```python
from build123d import *

# Parameters (mm, degrees)
F0_W     = 203.2
F0_H     = 203.2
F1_DEPTH = 9.525
F3_DEPTH = 76.2
F4_W     = 38.1
F4_H     = 63.5
F5_DEPTH = 101.6
F6_W     = 101.6
F6_H     = 190.5
F6_H_2   = 152.4
F7_DEPTH = 53.975


with BuildPart() as f1:
    # F0 (on Front) → F1 (new body, symmetric)
    with BuildSketch(Plane.XZ):
        Rectangle(F0_W, F0_H)
    extrude(amount=F1_DEPTH, both=True)

    # F2 (on Right) → F3 (join, symmetric)
    with BuildSketch(Plane.YZ):
        Polygon((-9.525, -101.6), (-9.525, 165.1), (-63.5, 165.1), (-63.5, 12.7), (-22.225, -101.6), align=None)
    extrude(amount=F3_DEPTH, both=True)

    # F4 (on Right) → F5 (cut, symmetric)
    with BuildSketch(Plane.YZ):
        with Locations((-9.525, 133.35)):
            Rectangle(F4_W, F4_H)
    extrude(amount=F5_DEPTH, both=True, mode=Mode.SUBTRACT)

    # F6 (on face) → F7 (cut, through all)
    with BuildSketch(Plane.XZ.offset(63.5)):
        with Locations((0, -82.55)):
            Rectangle(F6_W, F6_H)
        with Locations((0, 88.9)):
            Rectangle(F6_W, F6_H_2)
    extrude(amount=-F7_DEPTH, mode=Mode.SUBTRACT)


solid = f1.part
```
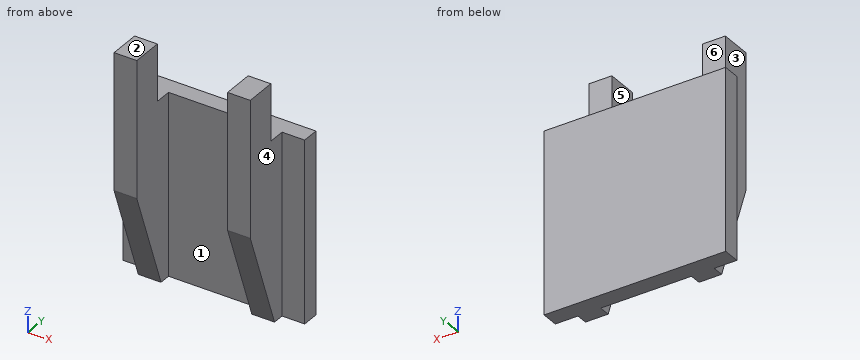
Source: CAD feature listing. Evaluate the final solid. Frame: model axes, mm. Face numbers are marked on the shaded views. A direction names the side the tool comes from. Round coordinates to 2 decimals unless told otherwise and drop trailing zeros. Write each loop counter-clockwise with the first axis right and the second up, starting at its lowest first coordinate (ties: lowest second). Pieces come first, ordered by that corner, then holes. Notation, with made-up numbers: M 42.25,-28.5 L 101.25,-28.5 A17 cw 101.25,-3.5 Z; hole C 5.5,0 d11. An arc over 180 degrees is marked long. Use CSV: the item, a comma, the result in double quotes. Start each with the question number.
Q1. Pull-direction query (X, two-part tool) for the marked faces 1, 2 and 3; classes: +X half, -X half, draft (parallel to the pull), parting line (faces both ways), or undercut.
Q2. Cut plane A-A on y = -15.5. Output: boundary loops of the cut face in (x, z), plus the area to 3 significant figures.
Q3. Line query: line 1 (X direction, y = -17.5, z = 33); line 2 (Y direction, x = 27, z = -9.5) (3 decimals); line 3 (Z direction, x = 50.5, y = -4). Output: solid intervals per line, ascending. Write a range as from..to.
Q4. Cut plane B-B on z = 44.5. Output: boundary loops of the cut face in (x, y) (3 decimals), plus the area to 3 significant figures.
Q5. Access query for the marked faces 4, 5 and 6. Directions: +Z, -Z, +X, -X, +Y, -Y. A direction counts if a zero-diameter tool reaches every point of the face in a straight line with its end or side. Return the directions, or none.
Q6. Cut plane C-C on x = -70. Output: boundary loops of the cut face in (y, z) (3 decimals), plus the area to 3 significant figures.
Q7. Cut plane D-D on y = -42. Output: boundary loops of the cut face in (x, z), plus the area to 3 significant figures.
Q8. First-contact query: P1, Ø16, axis at y = -33, z = 52.5, coming from the -X side; P2, Ø12.5, axis at x = 90.5, z = -46.5, coming from the -Y side (3 decimals); P3, Ø2, axis at y = -29, z = -38.5, coming from the +X side; P4, Ø11.5, axis at x = -19, y = -18, coming from the +Z side. Flat tips, straight axial feed; report the tip coordinate or a pass-through.
Results found:
1,face 1,"undercut"
1,face 2,"draft"
1,face 3,"-X half"
2,outline,"M -76.2,-101.6 L -50.8,-101.6 L -50.8,101.6 L -76.2,101.6 Z; M 50.8,-101.6 L 76.2,-101.6 L 76.2,101.6 L 50.8,101.6 Z"
2,area,"10,300 mm^2"
3,line 1,"-76.2..-50.8, 50.8..76.2"
3,line 2,"-9.525..9.525"
3,line 3,"-101.6..101.6"
4,outline,"M -101.6,-9.525 L -76.2,-9.525 L -76.2,-63.5 L -50.8,-63.5 L -50.8,-9.525 L 50.8,-9.525 L 50.8,-63.5 L 76.2,-63.5 L 76.2,-9.525 L 101.6,-9.525 L 101.6,9.525 L -101.6,9.525 Z"
4,area,"6,610 mm^2"
5,face 4,"+Z, -Z, +X, -Y"
5,face 5,"+Z, -Z, -Y"
5,face 6,"+Z, +X, -X, +Y"
6,outline,"M -63.5,12.7 L -22.225,-101.6 L 9.525,-101.6 L 9.525,101.6 L -28.575,101.6 L -28.575,165.1 L -63.5,165.1 Z"
6,area,"14,700 mm^2"
7,outline,"M -76.2,-46.84 L -50.8,-46.84 L -50.8,165.1 L -76.2,165.1 Z; M 50.8,-46.84 L 76.2,-46.84 L 76.2,165.1 L 50.8,165.1 Z"
7,area,"10,800 mm^2"
8,P1,"x = -76.2"
8,P2,"y = -9.525"
8,P3,"x = 76.2"
8,P4,"through"
